Could you check a few things on this drawing? It's one solid part, dimensions in mm from its lowest x, y, z. A direction names the side the tool comes from. Coordinates: 2 decimals unless noted, no trailing zeros. Order: outer loops, then holes, each group sorted by start corner. A loop starts at its lowest first (then second) coordinate and runs counter-clockwise, first axis right, second up. Notation, with made-up numbers: (-24, 55) -> (9, 55) arc R12 cw to (9, 59) -> close; hole circle Ø11 at (56.5, -9.75). An arc over 180 degrees is marked (long way). Use a Markdown table: item, result. Add a question column.
1. Suppose I cut it at A-A, the plane z = 123.19. List the corners of the cut face in (x, y) for me (1 decimal).
2. If I drill on line 1 along Y through (x, z) = (2, 161.29); line 2 along Y through (x, z) = (3.5, 11) (3 decimals), over which ranges is the centre line in solid material (lowest first)? Write a range as from..to.
3. For the marked faces 1 and 2, which set-ups out of +Z, -Z, +X, -X, +Y, -Y let a thin tool reach every point of the face, with its end or its side?
4. Suppose I cut it at B-B, the plane y = 25.4. List the corners of the cut face in (x, z) for me (1 decimal).
5. For pin 1 Ø4 at (y, z) = (32.5, 170) entering from +X; pin 2 Ø6 at (y, z) = (7, 146.5) entering from +X (3 decimals); pin 3 Ø12 at (x, z) = (10.5, 48) entering from +Y (3 decimals), each with a flat end and sliding along its axis, tell me the tip position at first contact or that it passes through.
6. Suppose I cut it at C-C, the plane z = 41. List the corners of the cut face in (x, y) for me (3 decimals).
7. Suppose I cut it at D-D, the plane y = 33. List the corners of the cut face in (x, z) for me (3 decimals), then the cut area to 3 significant figures.
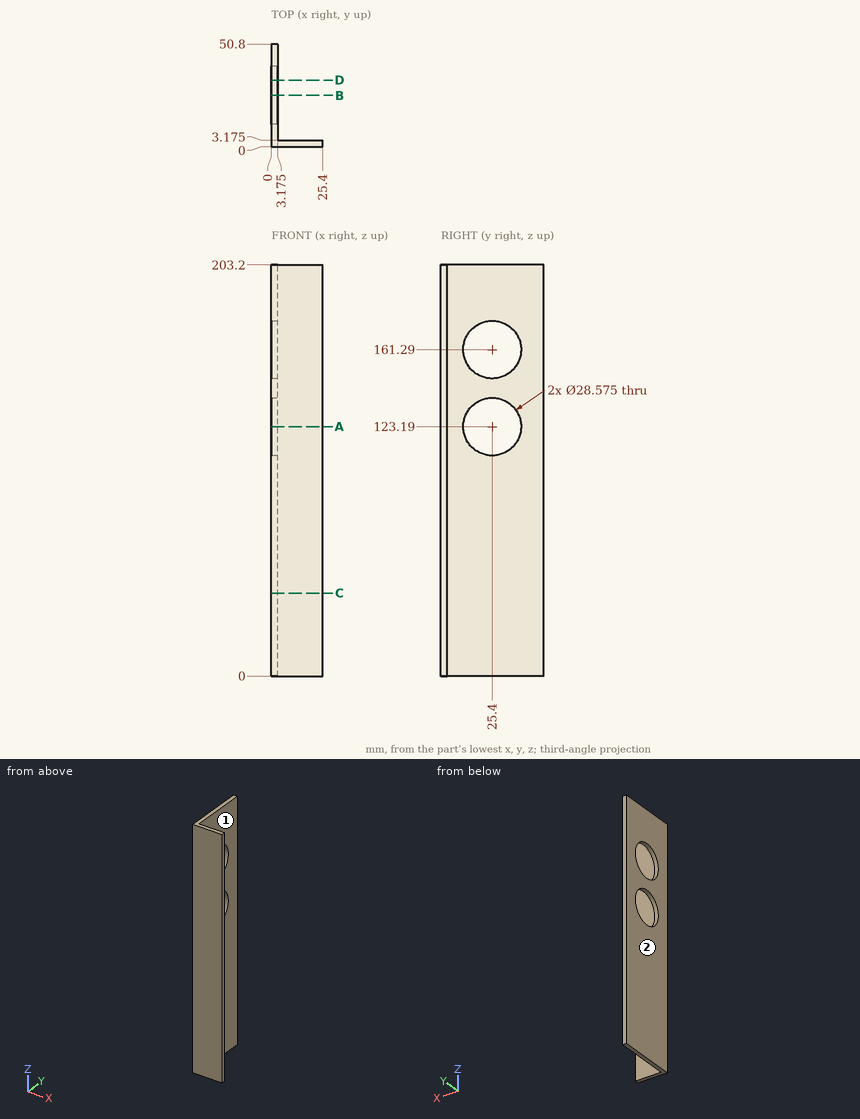
Worked out:
| question | item | result |
|---|---|---|
| 1 | outline | (0, 0) -> (25.4, 0) -> (25.4, 3.2) -> (3.2, 3.2) -> (3.2, 11.1) -> (0, 11.1) -> close; (0, 39.7) -> (3.2, 39.7) -> (3.2, 50.8) -> (0, 50.8) -> close |
| 2 | line 1 | y = 0..11.11, 39.69..50.8 |
| 2 | line 2 | y = 0..3.175 |
| 3 | face 1 | +Z, -Z, +X, +Y |
| 3 | face 2 | +Z, -Z, -X, +Y, -Y |
| 4 | outline | (0, 0) -> (3.2, 0) -> (3.2, 108.9) -> (0, 108.9) -> close; (0, 137.5) -> (3.2, 137.5) -> (3.2, 147) -> (0, 147) -> close; (0, 175.6) -> (3.2, 175.6) -> (3.2, 203.2) -> (0, 203.2) -> close |
| 5 | pin 1 | passes through |
| 5 | pin 2 | stops at x = 3.175 |
| 5 | pin 3 | stops at y = 3.175 |
| 6 | outline | (0, 0) -> (25.4, 0) -> (25.4, 3.175) -> (3.175, 3.175) -> (3.175, 50.8) -> (0, 50.8) -> close |
| 7 | outline | (0, 0) -> (3.175, 0) -> (3.175, 111.092) -> (0, 111.092) -> close; (0, 135.288) -> (3.175, 135.288) -> (3.175, 149.192) -> (0, 149.192) -> close; (0, 173.388) -> (3.175, 173.388) -> (3.175, 203.2) -> (0, 203.2) -> close |
| 7 | area | 492 mm² |
